CAD build for the part. Positions are in the model's coordinates, mm. Face numbers are marked on the shaded views. A direction names the side the tool comes from. Coordinates: 2 decimals unless noted, no trailing zeros. Order: outer loops, then holes, each group sorted by start corner. A loop starts at its lowest first (then second) coordinate and runs counter-clockwise, first axis right, second up. Notation, with made-up numbers: M 43,-25 L 54,-25 A24 cw 54,-14 Z; hole C 61.25,86 d4. An arc over 180 degrees is marked long. One line per item, written item: value.
from build123d import *

# Parameters (mm, degrees)
F1_DEPTH = 25.4
F2_W     = 23.985484906
F2_H     = 10.9293945134
F3_DEPTH = 63.5
F4_DEPTH = 67.31
F5_W     = 23.835350119
F5_H     = 2.447379753
F6_DEPTH = 66.04
F7_W     = 23.4697095584
F7_H     = 17.8560893983
F8_DEPTH = 34.29


# Not quite as in the source:
# - the program builds the solid bodies; features that only make, move or delete a surface that nothing else refers to are left out


with BuildPart() as f1:
    # F0 (on Right) → F1 (new body)
    with BuildSketch(Plane.YZ):
        Polygon((0, 0), (0, 3.2231518999), (-12.5630013645, 3.2231518999), (-20.3921347857, 3.2231518999), (-20.3921347857, 0), align=None)
        Polygon((-20.3921347857, 3.2231518999), (-12.5630013645, 3.2231518999), (-17.9742891341, 5.361024756), (-20.3921347857, 4.0822205165), align=None)
        with BuildLine():
            Line((-20.3921347857, 0), (-20.3921347857, 3.2231518999))
            Line((-20.3921347857, 3.2231518999), (-22.0163828564, 3.2231518999))
            ThreePointArc((-22.0163828564, 3.2231518999), (-22.7959834692, 3.2163945029), (-23.575584082, 3.2231518999))
            Line((-23.575584082, 3.2231518999), (-27.4015981704, 3.2231518999))
            Line((-27.4015981704, 3.2231518999), (-28.9092455059, 3.2231518999))
            Line((-28.9092455059, 3.2231518999), (-28.9092455059, 2.3980058104))
            Line((-28.9092455059, 2.3980058104), (-28.9092455059, 0))
            Line((-28.9092455059, 0), (-20.3921347857, 0))
        make_face()
        Polygon((-22.0163828564, 3.2231518999), (-20.3921347857, 3.2231518999), (-20.3921347857, 4.0822205165), align=None)
        with BuildLine():
            Line((-22.0454800874, 3.2231518999), (-22.0163828564, 3.2231518999))
            Line((-22.0163828564, 3.2231518999), (-20.3921347857, 4.0822205165))
            Line((-20.3921347857, 4.0822205165), (-20.3921347857, 20.491162315))
            ThreePointArc((-20.3921347857, 20.491162315), (-24.6506901458, 22.8198511271), (-28.9092455059, 20.491162315))
            Line((-28.9092455059, 20.491162315), (-28.9092455059, 3.6338099802))
            ThreePointArc((-28.9092455059, 3.6338099802), (-28.1561856735, 3.5369589297), (-27.4015981704, 3.4528343954))
            Line((-27.4015981704, 3.4528343954), (-27.4015981704, 18.5859873891))
            ThreePointArc((-27.4015981704, 18.5859873891), (-24.7235391289, 20.7198764309), (-22.0454800874, 18.5859873891))
            Line((-22.0454800874, 18.5859873891), (-22.0454800874, 3.2231518999))
        make_face()
        with BuildLine():
            ThreePointArc((-64.1917986715, 30.3313969183), (-50.16224019, 11.8027548597), (-28.9092455059, 2.3980058104))
            Line((-28.9092455059, 2.3980058104), (-28.9092455059, 3.2231518999))
            Line((-28.9092455059, 3.2231518999), (-28.9092455059, 3.6338099802))
            ThreePointArc((-28.9092455059, 3.6338099802), (-50.1126919116, 12.4626789581), (-64.1917986715, 30.6096847649))
            Line((-64.1917986715, 30.6096847649), (-64.1917986715, 30.3313969183))
        make_face()
        with BuildLine():
            Line((-28.9092455059, 3.2231518999), (-27.4015981704, 3.2231518999))
            Line((-27.4015981704, 3.2231518999), (-27.4015981704, 3.4528343954))
            ThreePointArc((-27.4015981704, 3.4528343954), (-28.1561856735, 3.5369589297), (-28.9092455059, 3.6338099802))
            Line((-28.9092455059, 3.6338099802), (-28.9092455059, 3.2231518999))
        make_face()
        with BuildLine():
            ThreePointArc((-67.6309564566, 44.6495479383), (-66.4828080231, 37.35321731), (-64.1917986715, 30.3313969183))
            Line((-64.1917986715, 30.3313969183), (-64.1917986715, 30.6096847649))
            ThreePointArc((-64.1917986715, 30.6096847649), (-64.3937854186, 31.0930746092), (-64.59012772, 31.5787844899))
            ThreePointArc((-64.59012772, 31.5787844899), (-65.5320044676, 34.1785482504), (-66.3123383407, 36.8312793835))
            ThreePointArc((-66.3123383407, 36.8312793835), (-66.4844767509, 37.5124245346), (-66.645954144, 38.1961755131))
            ThreePointArc((-66.645954144, 38.1961755131), (-66.7377613235, 38.6078575578), (-66.8257035474, 39.0203825019))
            ThreePointArc((-66.8257035474, 39.0203825019), (-67.3173861233, 41.8222257294), (-67.6309564566, 44.6495479383))
        make_face()
        with BuildLine():
            Line((-64.1917986715, 0), (-64.1917986715, 30.3313969183))
            ThreePointArc((-64.1917986715, 30.3313969183), (-66.4828080231, 37.35321731), (-67.6309564566, 44.6495479383))
            Line((-67.6309564566, 44.6495479383), (-67.6309564566, 0))
            Line((-67.6309564566, 0), (-64.1917986715, 0))
        make_face()
        with BuildLine():
            ThreePointArc((-64.59012772, 31.5787844899), (-64.3937854186, 31.0930746092), (-64.1917986715, 30.6096847649))
            Line((-64.1917986715, 30.6096847649), (-64.0304028831, 31.7278995465))
            Line((-64.0304028831, 31.7278995465), (-64.59012772, 31.5787844899))
        make_face()
        with BuildLine():
            Line((-64.0304028831, 31.7278995465), (-64.1917986715, 30.6096847649))
            Line((-64.1917986715, 30.6096847649), (-53.3271447245, 33.5041132079))
            ThreePointArc((-53.3271447245, 33.5041132079), (-50.3228913796, 38.4738529349), (-55.1768802106, 41.6617430747))
            Line((-55.1768802106, 41.6617430747), (-66.8257035474, 39.0203825019))
            ThreePointArc((-66.8257035474, 39.0203825019), (-66.7377613235, 38.6078575578), (-66.645954144, 38.1961755131))
            Line((-66.645954144, 38.1961755131), (-55.2403122474, 40.7000877275))
            ThreePointArc((-55.2403122474, 40.7000877275), (-51.4541715224, 38.3935253272), (-53.5909704186, 34.5090456743))
            Line((-53.5909704186, 34.5090456743), (-64.0304028831, 31.7278995465))
        make_face()
    extrude(amount=F1_DEPTH)

    # F2 (on Front) → F3 (cut)
    with BuildSketch(Plane.XZ):
        with Locations((12.7173874935, 37.006566301)):
            Rectangle(F2_W, F2_H)
    extrude(amount=F3_DEPTH, mode=Mode.SUBTRACT)

    # F2 (on Front) → F4 (cut)
    with BuildSketch(Plane.XZ):
        with Locations((12.7173874935, 37.006566301)):
            Rectangle(F2_W, F2_H)
    extrude(amount=F4_DEPTH, mode=Mode.SUBTRACT)

    # F5 (on Front) → F6 (cut)
    with BuildSketch(Plane.XZ):
        with Locations((12.7131266927, 31.5032089129)):
            Rectangle(F5_W, F5_H)
    extrude(amount=F6_DEPTH, mode=Mode.SUBTRACT)

    # F7 (on Front) → F8 (cut)
    with BuildSketch(Plane.XZ):
        with Locations((12.7604022855, 14.3902720883)):
            Rectangle(F7_W, F7_H)
    extrude(amount=F8_DEPTH, mode=Mode.SUBTRACT)


solid = f1.part
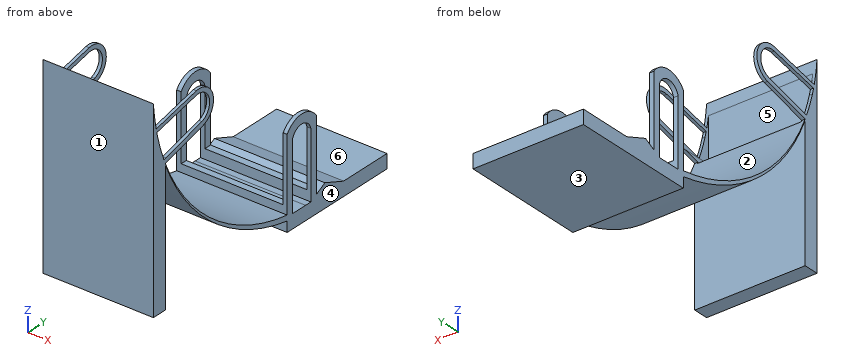
Q1. Slice it at B-B (z = 25). List the corners of the cut face in (x, y).
Recorded:
outline: M 0,-67.63 L 25.4,-67.63 L 25.4,-64.19 L 0,-64.19 Z; M 0,-61.56 L 25.4,-61.56 L 25.4,-61.33 L 0,-61.33 Z
Q2. Drill centre lines: line 1 along X through (y, z) = (-28, 17.5); line 2 along Y through (x, z) = (6.75, 37.5); line 3 along Z through (x, y) = (23, -28.5). Where is each one in solid material? Low to high.
Recorded:
line 1: x = 0 to 1.03, 24.5 to 25.4
line 2: y = -67.63 to -67.31
line 3: z = 0 to 5.46
Q3. Which spindle directions (+Z, -Z, +X, -X, +Y, -Y) get a long thin tool onto all of the face, cutting with end or side? Do the marked faces 4, 5 and 6. Say none if no direction does.
Recorded:
face 4: +Z, -Z, +X, +Y, -Y
face 5: +Z, +Y
face 6: +Z, +X, -X, +Y
Q4. Pin check, flat tips, straight feed: pin 1 Ø12 at (y, z) = (-33.5, 9.5) entering from +X; pin 2 Ø5 at (x, z) = (15.5, 13) entering from +Y; pin 3 Ø8 at (x, z) = (14.5, 18.5) entering from +Y; pin 4 Ø4 at (x, y) = (11.5, -8) entering from +Z. Stop position of each tip, or through.
Recorded:
pin 1: stops at x = 25.4
pin 2: stops at y = -47.33
pin 3: stops at y = -52.59
pin 4: stops at z = 3.22
Q5. Mould opens along Y. For the marked faces 1, 2 and 3 say: released by +Y, released by -Y, zero draft, split by the parting line, or undercut.
Recorded:
face 1: released by -Y
face 2: undercut
face 3: zero draft
Q6. Slice it at D-D (z = 7). List the corners of the cut face in (x, y), plus the area to 3 significant figures.
Recorded:
outline: M 0,-67.63 L 25.4,-67.63 L 25.4,-64.19 L 0,-64.19 Z; M 0,-42.74 L 25.4,-42.74 L 25.4,-40.85 L 0,-40.85 Z; M 0,-28.91 L 1.03,-28.91 L 1.03,-27.4 L 0,-27.4 Z; M 0,-22.05 L 1.03,-22.05 L 1.03,-20.39 L 0,-20.39 Z; M 24.5,-28.91 L 25.4,-28.91 L 25.4,-27.4 L 24.5,-27.4 Z; M 24.5,-22.05 L 25.4,-22.05 L 25.4,-20.39 L 24.5,-20.39 Z
area: 141 mm^2
Q7. Slice it at C-C (y = -56). List the corners of the cut face in (x, z).
Recorded:
outline: M 0,17.31 L 25.4,17.31 L 25.4,17.86 L 0,17.86 Z; M 0,32.79 L 0.72,32.79 L 0.72,33.87 L 0,33.87 Z; M 0,40.53 L 0.72,40.53 L 0.72,41.48 L 0,41.48 Z; M 24.71,32.79 L 25.4,32.79 L 25.4,33.87 L 24.71,33.87 Z; M 24.71,40.53 L 25.4,40.53 L 25.4,41.48 L 24.71,41.48 Z
